Can you work these out from the model? Positions are in its coordinate system, mm. Coordinates: 2 decimals unless noted, no trailing zeros. Order: outer loops, then holes, each group sorted by start corner. A loop starts at its lowest first (then second) coordinate and runs counter-clockwise, first axis right, second up. Notation, with made-up numbers: (52.5, 62.25) -> (74.5, 62.25) arc R35 cw to (74.5, 97.25) -> close; hole circle Ø5 at (-38, 39.25). An arc over 180 degrees is marked (long way). Return JSON: item names as keys, results as strings. Group by question number.
1) If I drill on probe 1 along Z at (x, y) = (-345.5, 44); probe 2 along X at (y, z) = (-21, 100); probe 3 along X at (y, z) = (33, 374.5), over which ranges is the centre line in solid material (lowest first)? Write a range as from..to.
2) If we section it at A-A, the plane y = 29: Please give me the cut outline in (x, z), then the cut area to 3 significant figures.
3) If we section it at B-B, the plane x = 387: Please give me the cut outline in (y, z).
4) For pin 1 (4 mm diameter, centred on y = -25, z = 361, fed in from -X); pin 2 (1 mm diameter, centred on y = -40, z = 187, fed in from -X); pin 3 (10 mm diameter, centred on x = 380, y = -37.5, fed in from +Z), each with a flat end and sliding along its axis, tell me the tip position at first contact or that it passes through.
5) If we section it at C-C, the plane z = 222.5: Please give me the cut outline in (x, y).
from build123d import *

# Parameters (mm, degrees)
F4_DEPTH = 53.34


# Not quite as in the source:
# - the program builds the solid bodies; features that only make, move or delete a surface that nothing else refers to are left out


with BuildPart() as f4:
    # F0 (on Front) → F4 (new body, symmetric)
    with BuildSketch(Plane.XZ):
        with BuildLine():
            Line((-548.9229032603, 53.3517466559), (-548.9229032603, 0))
            Line((-548.9229032603, 0), (517.8770967397, 0))
            Line((517.8770967397, 0), (517.8770967397, 53.3517466559))
            ThreePointArc((517.8770967397, 53.3517466559), (569.8826534338, 246.0368993204), (746.9217918528, 338.1742394829))
            Line((746.9217918528, 338.1742394829), (746.9217918528, 398.8678294032))
            ThreePointArc((746.9217918528, 398.8678294032), (533.7351343449, 346.9515616778), (414.162291011, 162.9782349944))
            ThreePointArc((414.162291011, 162.9782349944), (410.443214336, 139.7945515932), (408.564564689, 116.3897362155))
            ThreePointArc((408.564564689, 116.3897362155), (408.9628088542, 84.760149458), (412.718017276, 53.3517466559))
            Line((412.718017276, 53.3517466559), (111.3264834418, 53.3517466559))
            Line((111.3264834418, 53.3517466559), (78.2992156876, 53.3517466559))
            Line((78.2992156876, 53.3517466559), (0, 53.3517466559))
            Line((0, 53.3517466559), (-548.9229032603, 53.3517466559))
        make_face()
    extrude(amount=F4_DEPTH, both=True)


solid = f4.part
Result sheet:
{
 "1": {"probe 1": "z = 0..53.35", "probe 2": "x = 408.35..515.27", "probe 3": "x = 581.41..746.92"},
 "2": {"outline": "(-548.92, 0) -> (517.88, 0) -> (517.88, 53.35) arc R248.26 cw to (746.92, 338.17) -> (746.92, 398.87) arc R297.42 ccw to (412.72, 53.35) -> (-548.92, 53.35) -> close", "area": "103,000 mm2"},
 "3": {"outline": "(-53.34, 0) -> (53.34, 0) -> (53.34, 53.35) -> (-53.34, 53.35) -> close"},
 "4": {"pin 1": "stops at x = 552.14", "pin 2": "stops at x = 419.9", "pin 3": "stops at z = 53.35"},
 "5": {"outline": "(432.81, -53.34) -> (553.11, -53.34) -> (553.11, 53.34) -> (432.81, 53.34) -> close"}
}
